Source: CAD feature listing. Evaluate the final solid. Frame: model axes, mm. Coordinates: 2 decimals unless noted, no trailing zeros. Loops run counter-clockwise (first coordinate to the right, second up) from the corner with the lowest first, then second, coordinate; pieces in that order, holes last. Notation, with made-up numbers: M 71,27 L 116,27 A30 ccw 116,62 Z; hole C 80,-33.75 d5. An arc over 180 degrees is marked long. One line per question, with ' | ' between items. Start each with the question number.
1. Pin query (flat end, axial travel): P1, Ø3, axis at x = 1, z = -1.5, coming from the +Y side. Return the tip coordinate at first contact, or that it passes through.
2. Ray query, probe 1 along X at (y, z) = (0.05, 1.75); probe 2 along Y at (x, z) = (1.25, 6.25); probe 3 along Y at (x, z) = (-4.5, -6). Return the intervals inside material, ascending.
3. Section query A-A, the plane z = 0.75. Output: boundary loops of the cut face in (x, y) (3 decimals), and give its area (3 significant figures).
4. Section query B-B, the plane x = 0.5. Output: boundary loops of the cut face in (y, z), and give its area (3 significant figures).
```python
from build123d import *

# Parameters (mm, degrees)
ESQUISSE1_R                = 0.45
BOSS_EXTRU_1_DEPTH         = 7.5
R_P_TITION_LIN_AIRE1_COUNT = 8
R_P_TITION_LIN_AIRE1_PITCH = 1.27
BOSS_EXTRU_2_DEPTH         = 7.5
R_P_TITION_LIN_AIRE2_COUNT = 7
R_P_TITION_LIN_AIRE2_PITCH = 1.27


with BuildPart() as part:
    # Esquisse1 → Boss.-Extru.1 (new, symmetric)
    with BuildSketch(Plane.XY):
        with Locations((-4.445, 0)):
            Circle(ESQUISSE1_R)
    extrude(amount=BOSS_EXTRU_1_DEPTH, both=True)


with BuildPart() as r_p_tition_lin_aire1_1:
    # R_p_tition lin_aire1: pattern copy
    add(part.part.moved(Location(Vector(1, 0, 0) * (1 * R_P_TITION_LIN_AIRE1_PITCH))))


with BuildPart() as r_p_tition_lin_aire1_2:
    # R_p_tition lin_aire1: pattern copy
    add(part.part.moved(Location(Vector(1, 0, 0) * (2 * R_P_TITION_LIN_AIRE1_PITCH))))


with BuildPart() as r_p_tition_lin_aire1_3:
    # R_p_tition lin_aire1: pattern copy
    add(part.part.moved(Location(Vector(1, 0, 0) * (3 * R_P_TITION_LIN_AIRE1_PITCH))))


with BuildPart() as r_p_tition_lin_aire1_4:
    # R_p_tition lin_aire1: pattern copy
    add(part.part.moved(Location(Vector(1, 0, 0) * (4 * R_P_TITION_LIN_AIRE1_PITCH))))


with BuildPart() as r_p_tition_lin_aire1_5:
    # R_p_tition lin_aire1: pattern copy
    add(part.part.moved(Location(Vector(1, 0, 0) * (5 * R_P_TITION_LIN_AIRE1_PITCH))))


with BuildPart() as r_p_tition_lin_aire1_6:
    # R_p_tition lin_aire1: pattern copy
    add(part.part.moved(Location(Vector(1, 0, 0) * (6 * R_P_TITION_LIN_AIRE1_PITCH))))


with BuildPart() as r_p_tition_lin_aire1_7:
    # R_p_tition lin_aire1: pattern copy
    add(part.part.moved(Location(Vector(1, 0, 0) * (7 * R_P_TITION_LIN_AIRE1_PITCH))))


with BuildPart() as part_1:
    add(part.part)

    add(r_p_tition_lin_aire1_1.part)  # Boss.-Extru.2 merges R_p_tition lin_aire1_1
    # Esquisse2 → Boss.-Extru.2 (add, symmetric)
    with BuildSketch(Plane.XY):
        with BuildLine():
            Line((-4.006251781, 0.1), (-3.613748219, 0.1))
            ThreePointArc((-3.613748219, 0.1), (-3.625, 0), (-3.613748219, -0.1))
            Line((-3.613748219, -0.1), (-4.006251781, -0.1))
            ThreePointArc((-4.006251781, -0.1), (-3.995, 0), (-4.006251781, 0.1))
        make_face()
    boss_extru_2 = extrude(amount=BOSS_EXTRU_2_DEPTH, both=True)

    add(r_p_tition_lin_aire1_2.part)  # R_p_tition lin_aire2 merges R_p_tition lin_aire1_2

    add(r_p_tition_lin_aire1_3.part)  # R_p_tition lin_aire2 merges R_p_tition lin_aire1_3

    add(r_p_tition_lin_aire1_4.part)  # R_p_tition lin_aire2 merges R_p_tition lin_aire1_4

    add(r_p_tition_lin_aire1_5.part)  # R_p_tition lin_aire2 merges R_p_tition lin_aire1_5

    add(r_p_tition_lin_aire1_6.part)  # R_p_tition lin_aire2 merges R_p_tition lin_aire1_6

    add(r_p_tition_lin_aire1_7.part)  # R_p_tition lin_aire2 merges R_p_tition lin_aire1_7
    # R_p_tition lin_aire2: Boss.-Extru.2 ×7
    with Locations(*[(i * R_P_TITION_LIN_AIRE2_PITCH, 0, 0) for i in range(1, R_P_TITION_LIN_AIRE2_COUNT)]):
        add(boss_extru_2)


solid = part_1.part
```
Taken from the geometry:
1) P1: y = 0.45
2) probe 1: -4.89 to 4.89 | probe 2: -0.1 to 0.1 | probe 3: -0.45 to 0.45
3) outline: M -4.006,-0.1 L -3.614,-0.1 A0.45 ccw -2.736,-0.1 L -2.344,-0.1 A0.45 ccw -1.466,-0.1 L -1.074,-0.1 A0.45 ccw -0.196,-0.1 L 0.196,-0.1 A0.45 ccw 1.074,-0.1 L 1.466,-0.1 A0.45 ccw 2.344,-0.1 L 2.736,-0.1 A0.45 ccw 3.614,-0.1 L 4.006,-0.1 A0.45 ccw long 4.006,0.1 L 3.614,0.1 A0.45 ccw 2.736,0.1 L 2.344,0.1 A0.45 ccw 1.466,0.1 L 1.074,0.1 A0.45 ccw 0.196,0.1 L -0.196,0.1 A0.45 ccw -1.074,0.1 L -1.466,0.1 A0.45 ccw -2.344,0.1 L -2.736,0.1 A0.45 ccw -3.614,0.1 L -4.006,0.1 A0.45 ccw long Z | area: 5.62 mm^2
4) outline: M -0.43,-7.5 L 0.43,-7.5 L 0.43,7.5 L -0.43,7.5 Z | area: 12.9 mm^2
